Verification items for the finished model (mm, model axes). A direction names the side the tool comes from. Coordinates: 2 decimals unless noted, no trailing zeros. Order: outer loops, then holes, each group sorted by start corner. A loop starts at its lowest first (then second) coordinate and runs counter-clockwise, first axis right, second up.
Q1. Thickness scan on line 1 (X direction, y = -1, z = -70); line 2 (Y direction, x = -33, z = -117.5); line 3 (Y direction, x = 20.5, z = -77.5). Record the ranges inside material, lowest first.
Q2. Depth check by flat-ended pin: P1, Ø6, axis at y = 19.5, z = -25, coming from the +X side; P2, Ø4.5, axis at y = -1, z = -42.5, coming from the -X side; P3, Ø6, axis at y = 1, z = -124, coming from the -X side. Enter the tip coordinate at first touch or a pass-through.
Q3. Cross-section at B-B, the plane x = -23.5. Record the boundary of the cut face in (y, z), and give its area (3 significant figures).
Q4. Cross-section at C-C, the plane z = -58. Record the boundary of the cut face in (x, y), and give its area (3 significant figures).
Q5. Set-up check for faces 3 (the flat face through (-2, -13, -150)), 4 (the flat face through (3.68, 11.42, -73.95)): record each of +Z, -Z, +X, -X, +Y, -Y from which the full face is reachable in a straight line by a thin tool's end or side.
Q6. Draft check along Y on faces 1 (the flat face through (-2, -13, 0)), 2 (the flat face through (12, 0, -74)). Enter one of: pulls with the +Y half, pulls with the -Y half, needs draft (parallel to the pull), parting line crosses it, or undercut.
Q7. Cross-section at D-D, the plane x = 47. Record the boundary of the cut face in (y, z), and give its area (3 significant figures).
Q8. Cross-section at A-A, the plane y = 0. Record the boundary of the cut face in (x, z).
from build123d import *

# Parameters (mm, degrees)
BOSS_EXTRUDE1_DEPTH = 150
CUT_EXTRUDE1_DEPTH  = 177.988399984


with BuildPart() as part:
    # Sketch1 → Boss-Extrude1 (new body)
    with BuildSketch(Plane.XY):
        with BuildLine():
            ThreePointArc((34.172460266, -18.485243422), (69.5, 0), (34.172460266, 18.485243422))
            ThreePointArc((34.172460266, 18.485243422), (10.094920531, 17.484915258), (-1.077539734, 38.836840411))
            ThreePointArc((-1.077539734, 38.836840411), (-34.75, 60.188765563), (-33.094920531, 20.351596989))
            ThreePointArc((-33.094920531, 20.351596989), (-20.189841062, 0), (-33.094920531, -20.351596989))
            ThreePointArc((-33.094920531, -20.351596989), (-34.75, -60.188765563), (-1.077539734, -38.836840411))
            ThreePointArc((-1.077539734, -38.836840411), (10.094920531, -17.484915258), (34.172460266, -18.485243422))
        make_face()
    extrude(amount=-BOSS_EXTRUDE1_DEPTH)

    # Sketch2 → Cut-Extrude1 (cut, through all)
    with BuildSketch(Plane.XY):
        with BuildLine():
            Line((9.797958971, 2), (12, 2))
            Line((12, 2), (12, -2))
            Line((12, -2), (9.797958971, -2))
            ThreePointArc((9.797958971, -2), (8.090169944, -5.877852523), (4.929848865, -8.700378737))
            Line((4.929848865, -8.700378737), (5.610316965, -10.794644207))
            Line((5.610316965, -10.794644207), (1.8060909, -12.030712184))
            Line((1.8060909, -12.030712184), (1.1256228, -9.936446715))
            ThreePointArc((1.1256228, -9.936446715), (-3.090169944, -9.510565163), (-6.751144813, -7.377129775))
            Line((-6.751144813, -7.377129775), (-8.532633428, -8.671457016))
            Line((-8.532633428, -8.671457016), (-10.883774437, -5.435389039))
            Line((-10.883774437, -5.435389039), (-9.102285822, -4.141061797))
            ThreePointArc((-9.102285822, -4.141061797), (-10, 0), (-9.102285822, 4.141061797))
            Line((-9.102285822, 4.141061797), (-10.883774437, 5.435389039))
            Line((-10.883774437, 5.435389039), (-8.532633428, 8.671457016))
            Line((-8.532633428, 8.671457016), (-6.751144813, 7.377129775))
            ThreePointArc((-6.751144813, 7.377129775), (-3.090169944, 9.510565163), (1.1256228, 9.936446715))
            Line((1.1256228, 9.936446715), (1.8060909, 12.030712184))
            Line((1.8060909, 12.030712184), (5.610316965, 10.794644207))
            Line((5.610316965, 10.794644207), (4.929848865, 8.700378737))
            ThreePointArc((4.929848865, 8.700378737), (8.090169944, 5.877852523), (9.797958971, 2))
        make_face()
    extrude(amount=-CUT_EXTRUDE1_DEPTH, mode=Mode.SUBTRACT)


solid = part.part
Check values:
1. line 1: x = -20.21 to -9.95, 12 to 69.48
1. line 2: y = -61.1 to -20.31, 20.31 to 61.1
1. line 3: y = -14.49 to 14.49
2. P1: stops at x = 62.3
2. P2: stops at x = -20.43
2. P3: stops at x = -20.55
3. outline: (-63.2, -150) - (-11.75, -150) - (-11.75, 0) - (-63.2, 0) - close; (11.75, -150) - (63.2, -150) - (63.2, 0) - (11.75, 0) - close
3. area: 15,400 mm2
4. outline: (-33.09, -20.35) arc R22.5 ccw (long way) to (-1.08, -38.84) arc R22.5 cw to (34.17, -18.49) arc R22.5 ccw (long way) to (34.17, 18.49) arc R22.5 cw to (-1.08, 38.84) arc R22.5 ccw (long way) to (-33.09, 20.35) arc R22.5 cw to start; hole (-10.88, -5.44) - (-8.53, -8.67) - (-6.75, -7.38) arc R10 ccw to (1.13, -9.94) - (1.81, -12.03) - (5.61, -10.79) - (4.93, -8.7) arc R10 ccw to (9.8, -2) - (12, -2) - (12, 2) - (9.8, 2) arc R10 ccw to (4.93, 8.7) - (5.61, 10.79) - (1.81, 12.03) - (1.13, 9.94) arc R10 ccw to (-6.75, 7.38) - (-8.53, 8.67) - (-10.88, 5.44) - (-9.1, 4.14) arc R10 ccw to (-9.1, -4.14) - close
4. area: 6,450 mm2
5. face 3: -Z, +X, -X, +Y, -Y
5. face 4: +Z, -Z
6. face 1: needs draft
6. face 2: undercut
7. outline: (-22.5, -150) - (22.5, -150) - (22.5, 0) - (-22.5, 0) - close
7. area: 6,750 mm2
8. outline: (-20.19, -150) - (-10, -150) - (-10, 0) - (-20.19, 0) - close; (12, -150) - (69.5, -150) - (69.5, 0) - (12, 0) - close
